from build123d import *

# Parameters (mm, degrees)
BOX001_W     = 8
BOX001_H     = 8
BOX001_DEPTH = 3
BOX_W        = 10.2
BOX_H        = 10.2
BOX_DEPTH    = 3.9
FILLET_R     = 0.5


with BuildPart() as cube001:
    # Box001 → Box001 (new body)
    with BuildSketch(Plane(origin=(-4, -4, 0), x_dir=(1, 0, 0), z_dir=(0, 0, 1))):
        with Locations((4, 4)):
            Rectangle(BOX001_W, BOX001_H)
    extrude(amount=BOX001_DEPTH)


with BuildPart() as fillet_body:
    # Box → Box (new body)
    with BuildSketch(Plane(origin=(-5.1, -5.1, 0), x_dir=(1, 0, 0), z_dir=(0, 0, 1))):
        with Locations((5.1, 5.1)):
            Rectangle(BOX_W, BOX_H)
    extrude(amount=BOX_DEPTH)

    # Cut: cut Cube001
    add(cube001.part, mode=Mode.SUBTRACT)

    # Fillet
    fillet_edges = [fillet_body.edges().sort_by_distance(p)[0] for p in [
        (-5.1, 0, 3.9),
        (0, -5.1, 3.9),
        (0, 5.1, 3.9),
        (5.1, 0, 3.9),
    ]]
    fillet(fillet_edges, radius=FILLET_R)


solid = fillet_body.part
Could you check a few things on this model? Use its own coordinates, in mm. A direction names the side the tool comes from. Round coordinates to 2 decimals unless told otherwise and drop trailing zeros. Write each loop counter-clockwise with the first axis right and the second up, starting at its lowest first coordinate (ties: lowest second). Pieces come first, ordered by that corner, then holes. Notation, with made-up numbers: (12.25, 27.5) -> (42.25, 27.5) arc R15 ccw to (42.25, 56.5) -> close; hole circle Ø8 at (41, 60.25). An arc over 180 degrees is marked (long way). Use a Markdown table: item, result.
1. For pin 1 Ø3 at (x, y) = (-1, -1) entering from -Z, with a flat end and sliding along its axis, tell me the tip position at first contact or that it passes through.
Answer key:
| item | result |
|---|---|
| pin 1 | stops at z = 3 |
2. We'd pull the mould along X, two halves only. Please class faces 3 (the face through (0, -4, 1)), 4 (the face through (0, -5.1, 2)), 5 (the face through (5.1, 0, 2)): +X half, -X half, draft (parallel to the pull), parting line (faces both ways), or undercut.
Answer key:
| item | result |
|---|---|
| face 3 | undercut |
| face 4 | draft |
| face 5 | +X half |
3. If we section it at A-A (y = 2.5): List the corners of the cut face in (x, z) for me, then the cut area to 3 significant figures.
Answer key:
| item | result |
|---|---|
| outline | (-5.1, 0) -> (-4, 0) -> (-4, 3) -> (4, 3) -> (4, 0) -> (5.1, 0) -> (5.1, 3.4) arc R0.5 ccw to (4.6, 3.9) -> (-4.6, 3.9) arc R0.5 ccw to (-5.1, 3.4) -> close |
| area | 15.7 mm^2 |
4. Which directions (+Z, -Z, +X, -X, +Y, -Y) give clear straight access to the entire face, cutting with the end or side of a thin tool? Please do faces 1 (the face through (-4, 0, 1)), 2 (the face through (0, 5.1, 2)).
Answer key:
| item | result |
|---|---|
| face 1 | -Z |
| face 2 | +Z, -Z, +X, -X, +Y |
5. Please list where these lines run through material, in increasing order: probe 1 along Y at (x, z) = (3.25, 0.3); probe 2 along Z at (x, y) = (-3.5, -3.75).
Answer key:
| item | result |
|---|---|
| probe 1 | y = -5.1 to -4, 4 to 5.1 |
| probe 2 | z = 3 to 3.9 |
6. If we section it at B-B (z = 0.95): List the corners of the cut face in (x, y) for me, then the cut area to 3 significant figures.
Answer key:
| item | result |
|---|---|
| outline | (-5.1, -5.1) -> (5.1, -5.1) -> (5.1, 5.1) -> (-5.1, 5.1) -> close; hole (-4, -4) -> (4, -4) -> (4, 4) -> (-4, 4) -> close |
| area | 40.0 mm^2 |
